Can you work these out from the model? Positions are in its coordinate system, mm. Round coordinates to 2 decimals unless told otherwise and drop trailing zeros.
Q1. If we section it at A-A (y = 10.25): Count the separate pieces of the cut face and the enclosed holes in it, plus the area to 3 significant figures.
Q2. Will these pins go through, and if not, where does the flat tip stop? P1, Ø4, axis at x = -126.21, z = 83.79, coming from the +Y side; P2, Ø8, axis at x = 16.5, z = 92, coming from the -Y side.
Q3. If I drill on line 1 (Z direction, x = -126, y = 0.5); line 2 (Z direction, x = -126.5, y = 12.5), over which ranges is the centre line in solid material (lowest first)?
from build123d import *

# Parameters (mm, degrees)
SKETCH1_W           = 300
SKETCH1_H           = 300
BOSS_EXTRUDE1_DEPTH = 15
SKETCH3_R           = 2.5
CUT_EXTRUDE1_DEPTH  = 16
FILLET1_R           = 40


with BuildPart() as part:
    # Sketch1 → Boss-Extrude1 (new body)
    with BuildSketch(Plane(origin=(0, 0, 0), x_dir=(1, 0, 0), z_dir=(0, 1, 0))):
        Rectangle(SKETCH1_W, SKETCH1_H)
    extrude(amount=BOSS_EXTRUDE1_DEPTH)

    # Sketch3 → Cut-Extrude1 (cut, through all)
    with BuildSketch(Plane(origin=(0, 15, 0), x_dir=(1, 0, 0), z_dir=(0, 1, 0))):
        with Locations((-83.786796564, 126.213203436)):
            Circle(SKETCH3_R)
        with Locations((-126.213203436, 83.786796564)):
            Circle(SKETCH3_R)
        with Locations((126.213203436, 83.786796564)):
            Circle(SKETCH3_R)
        with Locations((83.786796564, 126.213203436)):
            Circle(SKETCH3_R)
        with Locations((83.786796564, -126.213203436)):
            Circle(SKETCH3_R)
        with Locations((126.213203436, -83.786796564)):
            Circle(SKETCH3_R)
        with Locations((-126.213203436, -83.786796564)):
            Circle(SKETCH3_R)
        with Locations((-83.786796564, -126.213203436)):
            Circle(SKETCH3_R)
    extrude(amount=-CUT_EXTRUDE1_DEPTH, mode=Mode.SUBTRACT)

    # Fillet1
    fillet1_edges = [part.edges().sort_by_distance(p)[0] for p in [
        (150, 7.5, 150),
        (-150, 7.5, 150),
        (-150, 7.5, -150),
        (150, 7.5, -150),
    ]]
    fillet(fillet1_edges, radius=FILLET1_R)


solid = part.part
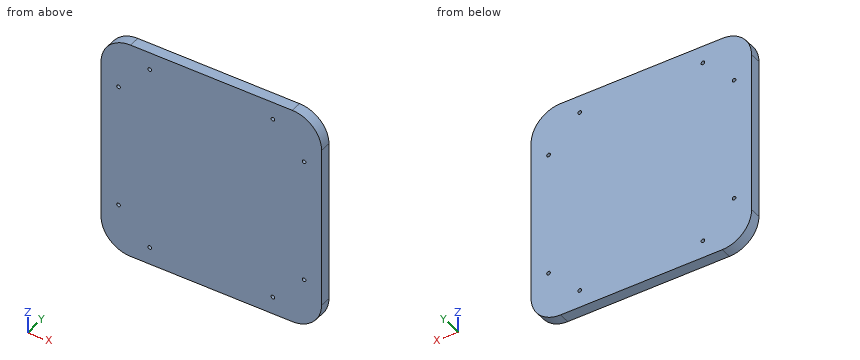
Solution:
1. separate pieces: 1
1. enclosed holes: 8
1. area: 88,500 mm2
2. P1: passes through
2. P2: stops at y = 0
3. line 1: z = -146.66 to -86.28, -81.3 to 81.3, 86.28 to 146.66
3. line 2: z = -146.44 to -86.27, -81.3 to 81.3, 86.27 to 146.44
